The model under review builds one solid part; all positions refer to its coordinate system, in mm. Give positions to 0.01 mm unless a question says otherwise; leave off trailing zeros. Write each loop counter-clockwise with the first axis right and the second up, starting at its lowest first coordinate (ties: lowest second). Pieces come first, ordered by that corner, then holes. Notation, with made-up numbers: (-2.5, 19) - (34.5, 19) arc R20 cw to (34.5, 41) - close; hole circle Ø5 at (-7, 51.25). An arc over 180 degrees is marked (long way). Write item = value, one per line.
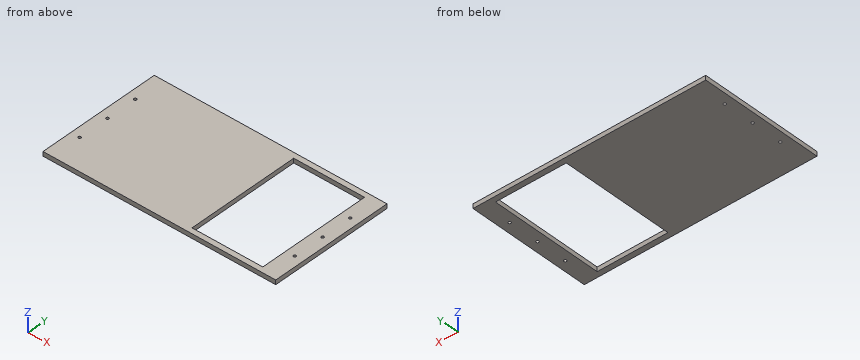
```python
from build123d import *

# Parameters (mm, degrees)
SKETCH_1_W      = 263
SKETCH_1_H      = 140
SKETCH_1_R      = 1.5
SKETCH_1_W_2    = 80
SKETCH_1_H_2    = 128
EXTRUDE_1_DEPTH = 5


with BuildPart() as part:
    # 草图1 → 凸台-拉伸1 (new body)
    with BuildSketch(Plane.XY):
        Rectangle(SKETCH_1_W, SKETCH_1_H)
        with Locations((-121.5, 35)):
            Circle(SKETCH_1_R, mode=Mode.SUBTRACT)
        with Locations((-121.5, 0)):
            Circle(SKETCH_1_R, mode=Mode.SUBTRACT)
        with Locations((-121.5, -35)):
            Circle(SKETCH_1_R, mode=Mode.SUBTRACT)
        with Locations(Location((121.5, -35, 0), (0, 0, 180))):
            Circle(SKETCH_1_R, mode=Mode.SUBTRACT)
        with Locations(Location((121.5, 0, 0), (0, 0, 180))):
            Circle(SKETCH_1_R, mode=Mode.SUBTRACT)
        with Locations(Location((121.5, 35, 0), (0, 0, 180))):
            Circle(SKETCH_1_R, mode=Mode.SUBTRACT)
        with Locations((71.5, 0)):
            Rectangle(SKETCH_1_W_2, SKETCH_1_H_2, mode=Mode.SUBTRACT)
    extrude(amount=EXTRUDE_1_DEPTH)


solid = part.part
```
1. For line 1 (Y direction, x = 121.5, z = 1.55); line 2 (X direction, y = -32, z = 0.45); line 3 (X direction, y = 0.5, z = 2.3), list the stretches that pass through material, from the lowest coordinate up. Write a range as from..to.
Findings below:
line_1 = -70..-36.5, -33.5..-1.5, 1.5..33.5, 36.5..70
line_2 = -131.5..31.5, 111.5..131.5
line_3 = -131.5..-122.91, -120.09..31.5, 111.5..120.09, 122.91..131.5
2. Take a section at B-B on y = 19.5. Give the boundary of the cut face in (x, z), and give its area (3 significant figures).
Findings below:
outline = (-131.5, 0) - (31.5, 0) - (31.5, 5) - (-131.5, 5) - close; (111.5, 0) - (131.5, 0) - (131.5, 5) - (111.5, 5) - close
area = 915 mm²
3. Insertion check: P1, Ø1.8, axis at x = 121.5, y = 35, coming from the +Z side. The pin has a flat end and moves straight along its axis. Give the tip position at first contact, or say it passes through.
Findings below:
P1 = through
4. Take a section at C-C on z = 3.45. Give the boundary of the cut face in (x, y).
Findings below:
outline = (-131.5, -70) - (131.5, -70) - (131.5, 70) - (-131.5, 70) - close; hole circle Ø3 at (-121.5, -35); hole circle Ø3 at (-121.5, 0); hole circle Ø3 at (-121.5, 35); hole (31.5, -64) - (111.5, -64) - (111.5, 64) - (31.5, 64) - close; hole circle Ø3 at (121.5, -35); hole circle Ø3 at (121.5, 0); hole circle Ø3 at (121.5, 35)
5. Take a section at A-A on x = 77.5. Give the boundary of the cut face in (y, z).
Findings below:
outline = (-70, 0) - (-64, 0) - (-64, 5) - (-70, 5) - close; (64, 0) - (70, 0) - (70, 5) - (64, 5) - close
